Model file for the job. Use its own axes, mm. Coordinates: 2 decimals unless noted, no trailing zeros. Order: outer loops, then holes, each group sorted by start corner. A loop starts at its lowest first (then second) coordinate and runs counter-clockwise, first axis right, second up.
from build123d import *

# Parameters (mm, degrees)
SKETCH_1_W          = 90.3
SKETCH_1_H          = 37
EXTRUDE_1_DEPTH     = 1.6
SKETCH_3_R          = 1.5
CUT_EXTRUDE_1_DEPTH = 1.6
SKETCH_4_W          = 6.3
SKETCH_4_H          = 8.293497289
EXTRUDE_2_DEPTH     = 7


with BuildPart() as part:
    # 草图1 → 凸台-拉伸1 (new body)
    with BuildSketch(Plane(origin=(0, 0, 0), x_dir=(1, 0, 0), z_dir=(0, 1, 0))):
        Rectangle(SKETCH_1_W, SKETCH_1_H)
    extrude(amount=EXTRUDE_1_DEPTH)

    # 草图3 → 切除-拉伸1 (cut)
    with BuildSketch(Plane(origin=(0, 1.6, 0), x_dir=(1, 0, 0), z_dir=(0, 1, 0))):
        with Locations(Location((0, -6, 0), (0, 0, 270))):
            Circle(SKETCH_3_R)
        with BuildLine():
            Line((-31.238672513, -7.65), (-53.101992088, -7.65))
            ThreePointArc((-53.101992088, -7.65), (-54.751992088, -6), (-53.101992088, -4.35))
            Line((-53.101992088, -4.35), (-31.238672513, -4.35))
            ThreePointArc((-31.238672513, -4.35), (-29.588672513, -6), (-31.238672513, -7.65))
        make_face()
        with BuildLine():
            Line((-24.944724021, -4.35), (-9.244724021, -4.35))
            ThreePointArc((-9.244724021, -4.35), (-7.594724021, -6), (-9.244724021, -7.65))
            Line((-9.244724021, -7.65), (-24.944724021, -7.65))
            ThreePointArc((-24.944724021, -7.65), (-26.594724021, -6), (-24.944724021, -4.35))
        make_face()
        with BuildLine():
            Line((31.238672513, -7.65), (53.101992088, -7.65))
            ThreePointArc((53.101992088, -7.65), (54.751992088, -6), (53.101992088, -4.35))
            Line((53.101992088, -4.35), (31.238672513, -4.35))
            ThreePointArc((31.238672513, -4.35), (29.588672513, -6), (31.238672513, -7.65))
        make_face()
        with BuildLine():
            Line((24.944724021, -4.35), (9.244724021, -4.35))
            ThreePointArc((9.244724021, -4.35), (7.594724021, -6), (9.244724021, -7.65))
            Line((9.244724021, -7.65), (24.944724021, -7.65))
            ThreePointArc((24.944724021, -7.65), (26.594724021, -6), (24.944724021, -4.35))
        make_face()
    extrude(amount=-CUT_EXTRUDE_1_DEPTH, mode=Mode.SUBTRACT)

    # 草图4 → 凸台-拉伸2 (add)
    with BuildSketch(Plane(origin=(0, 1.6, 0), x_dir=(1, 0, 0), z_dir=(0, 1, 0))):
        with Locations((-30, 14.353251355)):
            Rectangle(SKETCH_4_W, SKETCH_4_H)
        with Locations((-42, 14.353251355)):
            Rectangle(SKETCH_4_W, SKETCH_4_H)
        with Locations((-18, 14.353251355)):
            Rectangle(SKETCH_4_W, SKETCH_4_H)
        with Locations((-6, 14.353251355)):
            Rectangle(SKETCH_4_W, SKETCH_4_H)
        with Locations((6, 14.353251355)):
            Rectangle(SKETCH_4_W, SKETCH_4_H)
        with Locations((18, 14.353251355)):
            Rectangle(SKETCH_4_W, SKETCH_4_H)
        with Locations((30, 14.353251355)):
            Rectangle(SKETCH_4_W, SKETCH_4_H)
        with Locations((42, 14.353251355)):
            Rectangle(SKETCH_4_W, SKETCH_4_H)
    extrude(amount=EXTRUDE_2_DEPTH)


solid = part.part
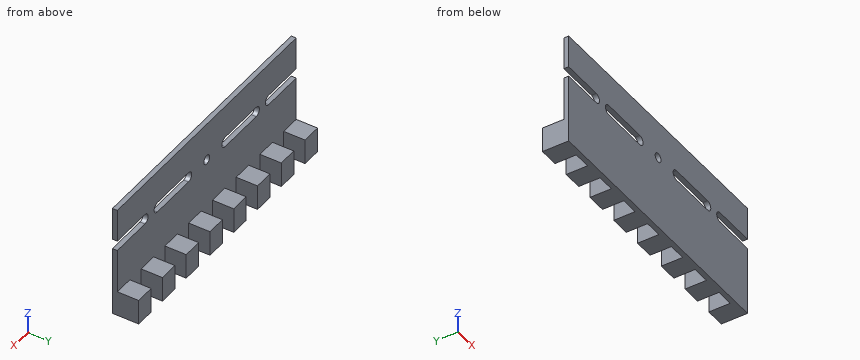
Q1. Cut at A-A, the plane y = 3.5. Count the separate pieces of the cut face and the enclosed holes in it, plus the area to 3 significant figures.
Established:
separate pieces: 8
enclosed holes: 0
area: 418 mm2
Q2. Cut at D-D, the plane x = -11.5. List the corners of the cut face in (y, z), plus the area to 3 significant figures.
Established:
outline: (0, -18.5) - (1.6, -18.5) - (1.6, 4.35) - (0, 4.35) - close; (0, 7.65) - (1.6, 7.65) - (1.6, 18.5) - (0, 18.5) - close
area: 53.9 mm2
Q3. Probe line 1 (X direction, y = 0.4, z = 6); line 2 (Y direction, x = 9, z = 11); line 3 (Z direction, x = -7, y = 2). List the from-to ranges inside material, lowest first.
Established:
line 1: x = -29.59 to -26.59, -7.59 to -1.5, 1.5 to 7.59, 26.59 to 29.59
line 2: y = 0 to 1.6
line 3: z = -18.5 to -10.21
Q4. Drop flat-ended pins along their axis: P1, Ø2, axis at x = 20.5, y = 4, coming from the +Z side; P2, Ø8, axis at x = 6, z = 11.5, coming from the +Y side. Give the stop position or say it passes through.
Established:
P1: stops at z = -10.21
P2: stops at y = 1.6
Q5. Cut at B-B, the plane z = 6. List the corners of the cut face in (x, y), plus the area to 3 significant figures.
Established:
outline: (-29.59, 0) - (-26.59, 0) - (-26.59, 1.6) - (-29.59, 1.6) - close; (-7.59, 0) - (-1.5, 0) - (-1.5, 1.6) - (-7.59, 1.6) - close; (1.5, 0) - (7.59, 0) - (7.59, 1.6) - (1.5, 1.6) - close; (26.59, 0) - (29.59, 0) - (29.59, 1.6) - (26.59, 1.6) - close
area: 29.1 mm2
Q6. Cut at C-C, the plane x = 0. List the corners of the cut face in (y, z), plus the area to 3 significant figures.
Established:
outline: (0, -18.5) - (1.6, -18.5) - (1.6, 4.5) - (0, 4.5) - close; (0, 7.5) - (1.6, 7.5) - (1.6, 18.5) - (0, 18.5) - close
area: 54.4 mm2
